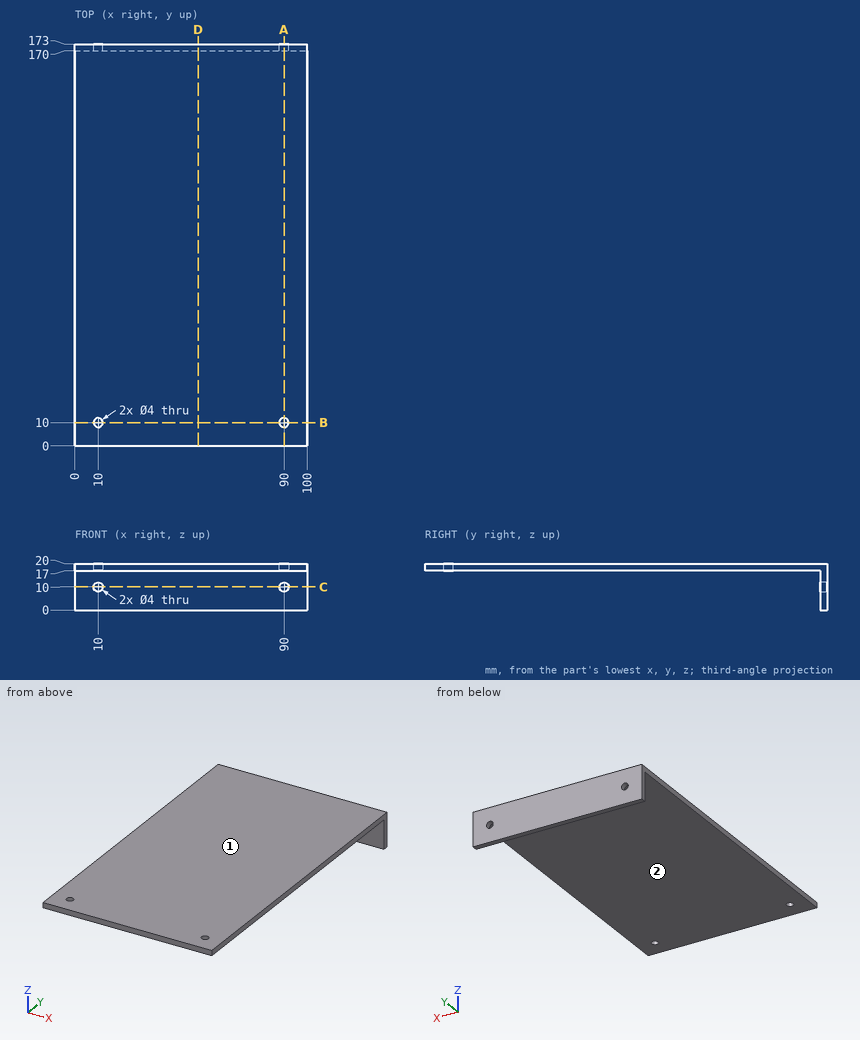
Source: three-view drawing plus pictorial views. Frame: mm from the lowest corner of the part. A direction names the side the tool comes from. Give positions to 0.01 mm unless a question says otherwise; leave off trailing zeros. Write each loop counter-clockwise with the first axis right and the second up, starting at its lowest first coordinate (ties: lowest second). Pieces come first, ordered by that corner, then holes.
(1) Access query for the marked faces 1 and 2. Directions: +Z, -Z, +X, -X, +Y, -Y. A direction counts if a zero-diameter tool reaches every point of the face in a straight line with its end or side. Return the directions, or none.
(2) Ray query, line 1 (X direction, y = 10, z = 17.85); line 2 (Y direction, x = 90, z = 18.9); line 3 (Z direction, x = 64.5, y = 147). Return the intervals inside material, ascending.
(3) Cut plane C-C, the plane z = 10. Return loops of the section in (x, y).
(4) Cut plane B-B, the plane y = 10. Return loops of the section in (x, z), then the cut area to 3 significant figures.
(5) First-contact query: P1, Ø1.5, axis at x = 21, y = 30, coming from the -Z side; P2, Ø2, axis at x = 78, z = 3.5, coming from the -Y side. Flat tips, straight axial feed; report the tip coordinate or a pass-through.
(6) Cut plane D-D, the plane x = 53. Return loops of the section in (y, z), then the cut area to 3 significant figures.
(7) Cut plane A-A, the plane x = 90. Return loops of the section in (y, z), then the cut area to 3 significant figures.
Values follow:
1. face 1: +Z, +X, -X, +Y, -Y
1. face 2: -Z, +X, -X, -Y
2. line 1: x = 0 to 8, 12 to 88, 92 to 100
2. line 2: y = 0 to 8, 12 to 173
2. line 3: z = 17 to 20
3. outline: (0, 170) - (8, 170) - (8, 173) - (0, 173) - close; (12, 170) - (88, 170) - (88, 173) - (12, 173) - close; (92, 170) - (100, 170) - (100, 173) - (92, 173) - close
4. outline: (0, 17) - (8, 17) - (8, 20) - (0, 20) - close; (12, 17) - (88, 17) - (88, 20) - (12, 20) - close; (92, 17) - (100, 17) - (100, 20) - (92, 20) - close
4. area: 276 mm2
5. P1: stops at z = 17
5. P2: stops at y = 170
6. outline: (0, 17) - (170, 17) - (170, 0) - (173, 0) - (173, 20) - (0, 20) - close
6. area: 570 mm2
7. outline: (0, 17) - (8, 17) - (8, 20) - (0, 20) - close; (12, 17) - (170, 17) - (170, 12) - (173, 12) - (173, 20) - (12, 20) - close; (170, 0) - (173, 0) - (173, 8) - (170, 8) - close
7. area: 546 mm2
